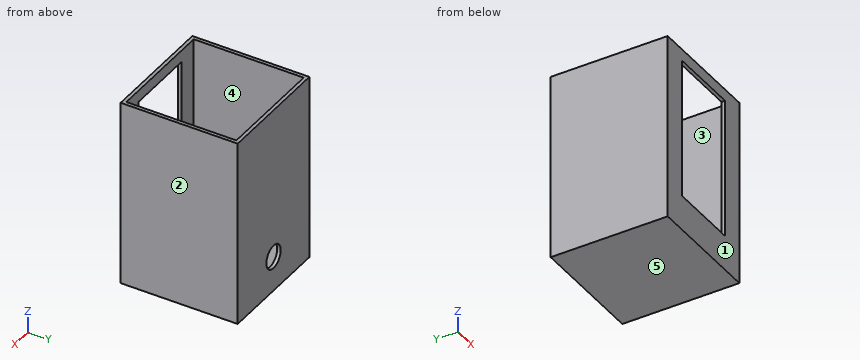
Autodesk Inventor part; units mm, degrees
ref_plane "YZ Plane" through (0, 0, 0) normal (1, 0, 0) x (0, 1, 0)
ref_plane "XZ Plane" through (0, 0, 0) normal (0, 1, 0) x (-1, 0, 0)
ref_plane "XY Plane" through (0, 0, 0) normal (0, 0, 1) x (1, 0, 0)
sketch "Esquisse2" plane through (0, 0, 0) normal (0, 0, 1) x (1, 0, 0)
  line L0 (-49.9248, 43.0827) -> (50.0752, 43.0827)
  line L1 (50.0752, 43.0827) -> (50.0752, -56.9173)
  line L2 (50.0752, -56.9173) -> (-49.9248, -56.9173)
  line L3 (-49.9248, -56.9173) -> (-49.9248, 43.0827)
  point P0 (0, 0)
  dimension "d0" = 100
  dimension "d1" = 100
extrude "Extrusion1" add sketch "Esquisse2" along normal blind 160
sketch "Esquisse3" plane through (0, 0, 160) normal (0, 0, 1) x (1, 0, 0)
  line L0 (-46.9248, 40.0827) -> (47.0752, 40.0827)
  line L1 (47.0752, 40.0827) -> (47.0752, -53.9173)
  line L2 (47.0752, -53.9173) -> (-46.9248, -53.9173)
  line L3 (-46.9248, -53.9173) -> (-46.9248, 40.0827)
  line L4 (50.0752, 43.0827) -> (-49.9248, 43.0827)
  line L5 (50.0752, -56.9173) -> (50.0752, 43.0827)
  line L6 (-49.9248, -56.9173) -> (50.0752, -56.9173)
  line L7 (-49.9248, 43.0827) -> (-49.9248, -56.9173)
  point P0 (0, 0)
  dimension "d4" = 3
  dimension "d5" = 3
  dimension "d6" = 3
  dimension "d7" = 3
extrude "Extrusion2" cut sketch "Esquisse3" against normal blind 155 contours L0 L1 L2 L3
sketch "Esquisse4" plane through (-49.9248, 43.0827, 0) normal (0, 1, 0) x (1, 0, 0)
  circle A0 centre (50, -30) radius 9.7582
  line L0 (100, 0) -> (100, -160)
  line L1 (100, 0) -> (0, 0)
  point P0 (49.9248, 0)
  dimension "d10" = 50
  dimension "d11" = 30
hole "Perçage1" at (0.0752, 43.0827, 30) direction (0, -1, 0) diameter 20 depth 8 tip angle 118
sketch "Esquisse5" plane through (-49.9248, -56.9173, 0) normal (0, -1, 0) x (1, 0, 0)
  line L0 (20, 150) -> (80, 150)
  line L1 (80, 150) -> (80, 30)
  line L2 (80, 30) -> (20, 30)
  line L3 (20, 30) -> (20, 150)
  line L4 (0, 0) -> (100, 0)
  line L5 (100, 0) -> (100, 160)
  point P0 (49.9248, 0)
  dimension "d19" = 60
  dimension "d20" = 120
  dimension "d21" = 30
  dimension "d22" = 20
extrude "Extrusion3" cut sketch "Esquisse5" against normal blind 5
properties part number "bloc station"
The model under review builds one solid part; all positions refer to its coordinate system, in mm. Face numbers are marked on the shaded views. A direction names the side the tool comes from. Round coordinates to 2 decimals unless told otherwise and drop trailing zeros. Write each loop counter-clockwise with the first axis right and the second up, starting at its lowest first coordinate (ties: lowest second). Pieces come first, ordered by that corner, then holes. Notation, with made-up numbers: (-37.5, 62) - (-16.5, 62) arc R25 ccw to (-16.5, 96) - close; hole circle Ø3 at (47, -37.75). An arc over 180 degrees is marked (long way). Answer as CSV lines item,"result". Start each with the question number.
(1) We need section B-B on y = -40. State the section outline as (x, z) points, plus the area to 3 significant figures.
(2) We need section D-D on z = 43. State the section outline as (x, y) points.
(3) Draft analysis for pull direction Y (two halves, no side actions). For the marked faces 1, 2 and 3, state which applies: pulls with the +Y half, pulls with the -Y half, needs draft (parallel to the pull), parting line crosses it, or undercut.
(4) To check wall thickness, follow line 1 (X direction, y = -43.5, z = 119); line 2 (Y direction, x = -34, z = 61); line 3 (X direction, y = 40.75, z = 30). State the ranges of each line that lie inside material, in increasing order.
(5) We need section C-C on x = -34.5. State the section outline as (y, z) points.
(6) We need section A-A on x = -16.5. State the section outline as (y, z) points, plus the area to 3 significant figures.
(7) For pin 1 Ø2 at (x, z) = (2.5, 136) entering from -Y, flat-tipped, find the tip position at first contact; note if it passes through.
(8) For the marked faces 4 and 5, list the 3-axis set-ups (+Z, -Z, +X, -X, +Y, -Y) from which the entire face can be reached by the end or side of a thin tool; tool diameter is ignored.
Worked answers:
1,outline,"(-49.92, 0) - (50.08, 0) - (50.08, 160) - (47.08, 160) - (47.08, 5) - (-46.92, 5) - (-46.92, 160) - (-49.92, 160) - close"
1,area,"1,430 mm²"
2,outline,"(-49.92, -56.92) - (-29.92, -56.92) - (-29.92, -53.92) - (-46.92, -53.92) - (-46.92, 40.08) - (47.08, 40.08) - (47.08, -53.92) - (30.08, -53.92) - (30.08, -56.92) - (50.08, -56.92) - (50.08, 43.08) - (-49.92, 43.08) - close"
3,face 1,"pulls with the -Y half"
3,face 2,"needs draft"
3,face 3,"undercut"
4,line 1,"-49.92 to -46.92, 47.08 to 50.08"
4,line 2,"-56.92 to -53.92, 40.08 to 43.08"
4,line 3,"-49.92 to -9.92, 10.08 to 50.08"
5,outline,"(-56.92, 0) - (43.08, 0) - (43.08, 160) - (40.08, 160) - (40.08, 5) - (-53.92, 5) - (-53.92, 160) - (-56.92, 160) - close"
6,outline,"(-56.92, 0) - (43.08, 0) - (43.08, 160) - (40.08, 160) - (40.08, 5) - (-53.92, 5) - (-53.92, 30) - (-56.92, 30) - close; (-56.92, 150) - (-53.92, 150) - (-53.92, 160) - (-56.92, 160) - close"
6,area,"1,070 mm²"
7,pin 1,"y = 40.08"
8,face 4,"+Z"
8,face 5,"-Z, +X, -X, +Y, -Y"
